```python
from build123d import *

# Parameters (mm, degrees)
ESQUISSE1_R             = 1.6
BOSS_EXTRU_1_DEPTH      = 3
ENL_V_MAT_EXTRU_1_DEPTH = 1.5
ESQUISSE4_W             = 13
ESQUISSE4_H             = 5
ENL_V_MAT_EXTRU_2_DEPTH = 26.511370014
CHANFREIN1_SIZE         = 2


with BuildPart() as part:
    # Esquisse1 → Boss.-Extru.1 (new body)
    with BuildSketch(Plane.XY):
        with BuildLine():
            Line((-9.5, 12.3), (9.5, 12.3))
            ThreePointArc((9.5, 12.3), (11.479898987, 11.479898987), (12.3, 9.5))
            Line((12.3, 9.5), (12.3, 8))
            ThreePointArc((12.3, 8), (13.2372583, 5.7372583), (15.5, 4.8))
            Line((15.5, 4.8), (19.5, 4.8))
            ThreePointArc((19.5, 4.8), (21.479898987, 3.979898987), (22.3, 2))
            Line((22.3, 2), (22.3, -2))
            ThreePointArc((22.3, -2), (21.479898987, -3.979898987), (19.5, -4.8))
            Line((19.5, -4.8), (15.5, -4.8))
            ThreePointArc((15.5, -4.8), (13.2372583, -5.7372583), (12.3, -8))
            Line((12.3, -8), (12.3, -9.5))
            ThreePointArc((12.3, -9.5), (11.479898987, -11.479898987), (9.5, -12.3))
            Line((9.5, -12.3), (-9.5, -12.3))
            ThreePointArc((-9.5, -12.3), (-11.479898987, -11.479898987), (-12.3, -9.5))
            Line((-12.3, -9.5), (-12.3, -8))
            ThreePointArc((-12.3, -8), (-13.2372583, -5.7372583), (-15.5, -4.8))
            Line((-15.5, -4.8), (-19.5, -4.8))
            ThreePointArc((-19.5, -4.8), (-21.479898987, -3.979898987), (-22.3, -2))
            Line((-22.3, -2), (-22.3, 2))
            ThreePointArc((-22.3, 2), (-21.479898987, 3.979898987), (-19.5, 4.8))
            Line((-19.5, 4.8), (-15.5, 4.8))
            ThreePointArc((-15.5, 4.8), (-13.2372583, 5.7372583), (-12.3, 8))
            Line((-12.3, 8), (-12.3, 9.5))
            ThreePointArc((-12.3, 9.5), (-11.479898987, 11.479898987), (-9.5, 12.3))
        make_face()
        with Locations((-17.5, 0)):
            Circle(ESQUISSE1_R, mode=Mode.SUBTRACT)
        with Locations((17.5, 0)):
            Circle(ESQUISSE1_R, mode=Mode.SUBTRACT)
    extrude(amount=BOSS_EXTRU_1_DEPTH)

    # Esquisse2 → Enlèv. mat.-Extru.1 (cut)
    with BuildSketch(Plane(origin=(0, 0, 0), x_dir=(-1, 0, 0), z_dir=(0, 0, -1))):
        with BuildLine():
            Line((-8.75, 11.75), (8.75, 11.75))
            ThreePointArc((8.75, 11.75), (10.871320344, 10.871320344), (11.75, 8.75))
            Line((11.75, 8.75), (11.75, -8.75))
            ThreePointArc((11.75, -8.75), (10.871320344, -10.871320344), (8.75, -11.75))
            Line((8.75, -11.75), (-8.75, -11.75))
            ThreePointArc((-8.75, -11.75), (-10.871320344, -10.871320344), (-11.75, -8.75))
            Line((-11.75, -8.75), (-11.75, 8.75))
            ThreePointArc((-11.75, 8.75), (-10.871320344, 10.871320344), (-8.75, 11.75))
        make_face()
    extrude(amount=-ENL_V_MAT_EXTRU_1_DEPTH, mode=Mode.SUBTRACT)

    # Esquisse4 → Enlèv. mat.-Extru.2 (cut, through all)
    with BuildSketch(Plane(origin=(0, 0, 1.5), x_dir=(-1, 0, 0), z_dir=(0, 0, -1))):
        with Locations((0, 6.25)):
            Rectangle(ESQUISSE4_W, ESQUISSE4_H)
        with Locations((0, -6.25)):
            Rectangle(ESQUISSE4_W, ESQUISSE4_H)
    extrude(amount=-ENL_V_MAT_EXTRU_2_DEPTH, mode=Mode.SUBTRACT)

    # Chanfrein1
    chanfrein1_edges = [part.edges().sort_by_distance(p)[0] for p in [
        (-19.1, 0, 3),
        (15.9, 0, 3),
    ]]
    chamfer(chanfrein1_edges, length=CHANFREIN1_SIZE)


solid = part.part
```
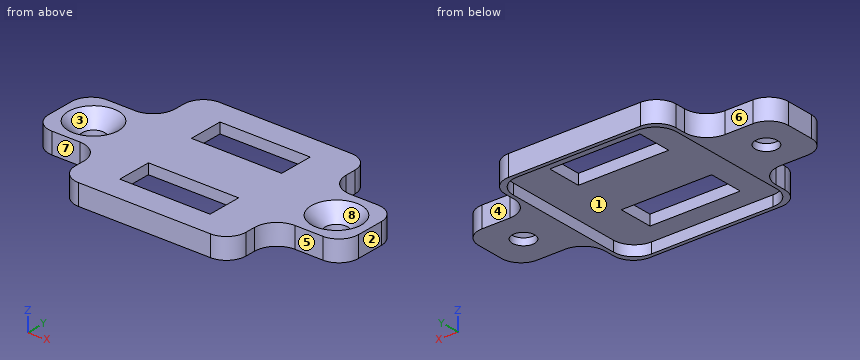
Geometry: final body of the model. Coordinates: model frame, mm. Face numbers are marked on the shaded views. A direction names the side the tool comes from. Round coordinates to 2 decimals unless told otherwise and drop trailing zeros. Write each loop counter-clockwise with the first axis right and the second up, starting at its lowest first coordinate (ties: lowest second). Pieces come first, ordered by that corner, then holes. Notation, with made-up numbers: (32.5, -2.75) -> (62.5, -2.75) arc R18 cw to (62.5, 7.25) -> close; hole circle Ø7 at (-6.75, 58.25). An arc over 180 degrees is marked (long way). Return JSON: item names as keys, results as strings.
Q1. Ray query, line 1 (Y direction, x = 3, z = 2.3); line 2 (Y direction, x = -17.5, z = 0.45); line 3 (X direction, y = -0.5, z = 1.45). Return the intervals inside material, ascending.
From the geometry:
{"line 1": "-12.3 to -8.75, -3.75 to 3.75, 8.75 to 12.3", "line 2": "-4.8 to -1.6, 1.6 to 4.8", "line 3": "-22.3 to -19.49, -15.51 to -11.75, 11.75 to 15.51, 19.49 to 22.3"}
Q2. First-contact query: pin 1 Ø1.6 at (y, z) = (-8.5, 1) entering from -X; pin 2 Ø8 at (x, y) = (-6, -0.5) entering from -Z; pin 3 Ø0.8 at (y, z) = (-6, 2) entering from +X; pin 4 Ø10 at (x, y) = (3.5, 7.5) entering from +Z. Flat tips, straight axial feed; report the tip coordinate or a pass-through.
From the geometry:
{"pin 1": "x = -12.31", "pin 2": "z = 1.5", "pin 3": "x = 13.38", "pin 4": "z = 3"}
Q3. Mould query, pull axis Y, two halves, no side actions, for the marked faces 1, 2, 3 and 4. Classes: +Y half, -Y half, draft (parallel to the pull), parting line (faces both ways), or undercut.
From the geometry:
{"face 1": "undercut", "face 2": "draft", "face 3": "undercut", "face 4": "+Y half"}
Q4. Section D-D on x = 5. Return the cut outline in (y, z), and give its area (4 significant figures).
From the geometry:
{"outline": "(-12.3, 0) -> (-11.75, 0) -> (-11.75, 1.5) -> (-8.75, 1.5) -> (-8.75, 3) -> (-12.3, 3) -> close; (-3.75, 1.5) -> (3.75, 1.5) -> (3.75, 3) -> (-3.75, 3) -> close; (8.75, 1.5) -> (11.75, 1.5) -> (11.75, 0) -> (12.3, 0) -> (12.3, 3) -> (8.75, 3) -> close", "area": "23.55 mm2"}
Q5. Section C-C on z = 2.1. Give the number of separate pieces and of enclosed holes in the cut face, and give its area (3 significant figures).
From the geometry:
{"separate pieces": "1", "enclosed holes": "4", "area": "617 mm2"}
Q6. Section A-A on x = 17.5. Return the cut outline in (y, z).
From the geometry:
{"outline": "(-4.8, 0) -> (-1.6, 0) -> (-1.6, 1) -> (-3.6, 3) -> (-4.8, 3) -> close; (1.6, 0) -> (4.8, 0) -> (4.8, 3) -> (3.6, 3) -> (1.6, 1) -> close"}
Q7. Section B-B on y = 0. Return the cut outline in (x, z), and give its area (4 significant figures).
From the geometry:
{"outline": "(-22.3, 0) -> (-19.1, 0) -> (-19.1, 1) -> (-21.1, 3) -> (-22.3, 3) -> close; (-15.9, 0) -> (-11.75, 0) -> (-11.75, 1.5) -> (11.75, 1.5) -> (11.75, 0) -> (15.9, 0) -> (15.9, 1) -> (13.9, 3) -> (-13.9, 3) -> (-15.9, 1) -> close; (19.1, 0) -> (22.3, 0) -> (22.3, 3) -> (21.1, 3) -> (19.1, 1) -> close", "area": "71.35 mm2"}
Q8. Set-up query: the marked faces 5, 6, 7 and 8. Return all of +Z, -Z, +X, -X, +Y, -Y with unobstructed straight access to the full face (end or side cutting, diameter ignored); none if empty.
From the geometry:
{"face 5": "+Z, -Z, +X, -Y", "face 6": "+Z, -Z, -X, +Y", "face 7": "+Z, -Z, -X, -Y", "face 8": "+Z"}
